Geometry check sheet. Reference: drawing and pictorial views, mm from the part's lowest x, y, z. A direction names the side the tool comes from. Coordinates: 2 decimals unless noted, no trailing zeros. Loops run counter-clockwise (first coordinate to the right, second up) from the corner with the lowest first, then second, coordinate; pieces in that order, holes last. Notation, with made-up numbers: (85, -23) - (139, -23) arc R16 ccw to (139, -10) - close; hole circle Ø11 at (16.5, -9.75). An arc over 180 degrees is marked (long way). Use a Markdown table: item, result. Add a question column.
1) Sectioned sample at A-A, the plane z = 7.75. Enter the section's corners in (x, y), then the cut area to 3 significant figures.
2) Thickness scan on line 1 (Y direction, x = 0.35, z = 8); line 2 (Z direction, x = 1.4, y = 17.75); line 3 (Z direction, x = 0.3, y = 5). Record the ranges inside material, lowest first.
3) Tool access check on the marked faces 1, 2, 3, 4 and 5. Record the directions out of +Z, -Z, +X, -X, +Y, -Y that give a thin tool (end or side, any length) a straight path to the whole face; none if there is none.
4) Go/stop test with flat-tipped pins: P1, Ø2.5, axis at x = 3.5, y = 14.5, coming from the -Z side; P2, Ø2.5, axis at x = 2, z = 12.5, coming from the -Y side. Record where each tip stops, or that it passes through.
5) Draft check along Y on the marked faces 6, 7 and 8. Enter one of: pulls with the +Y half, pulls with the -Y half, needs draft (parallel to the pull), parting line crosses it, or undercut.
6) Sectioned sample at D-D, the plane y = 5.25. Enter the section's corners in (x, z), then the cut area to 3 significant figures.
7) Sectioned sample at C-C, the plane z = 12.25. Enter the section's corners in (x, y).
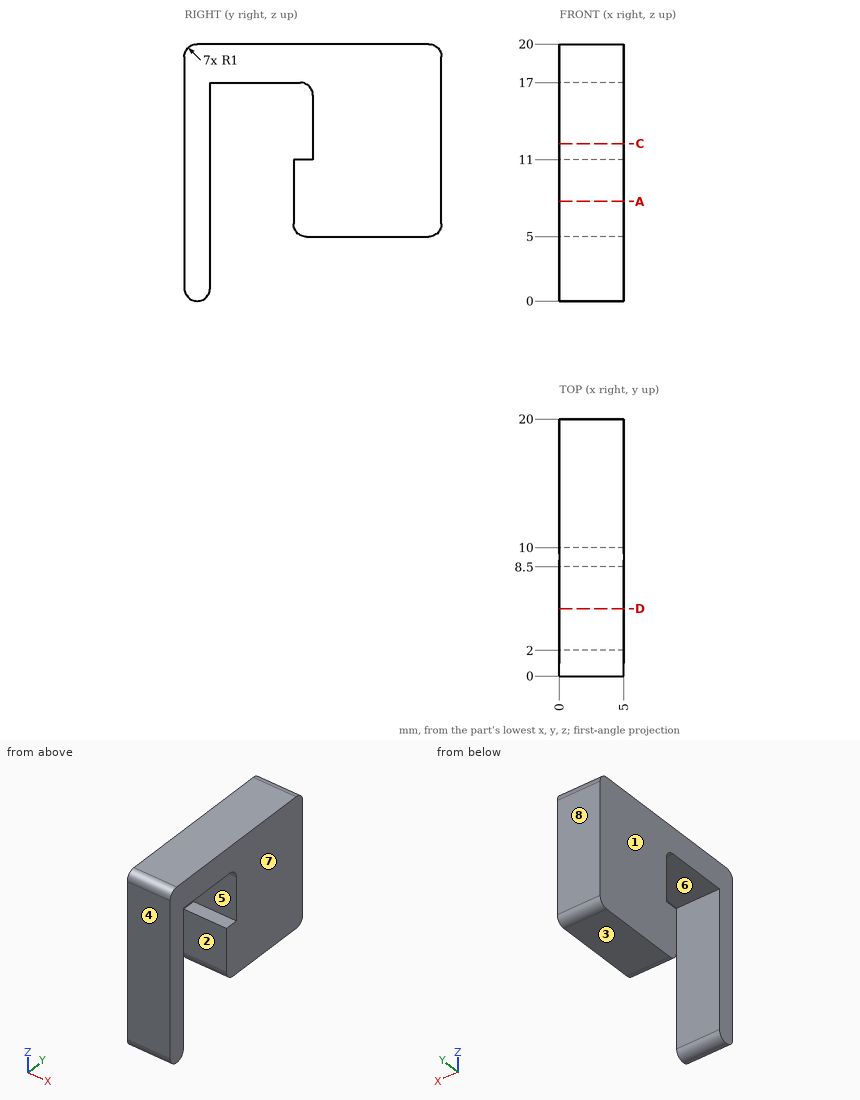
Solved:
| question | item | result |
|---|---|---|
| 1 | outline | (0, 0) - (5, 0) - (5, 2) - (0, 2) - close; (0, 8.5) - (5, 8.5) - (5, 20) - (0, 20) - close |
| 1 | area | 67.5 mm2 |
| 2 | line 1 | y = 0 to 2, 8.5 to 20 |
| 2 | line 2 | z = 5 to 20 |
| 2 | line 3 | z = 17 to 20 |
| 3 | face 1 | +Z, -Z, -X, +Y, -Y |
| 3 | face 2 | -Z, +X, -X |
| 3 | face 3 | -Z, +X, -X, +Y |
| 3 | face 4 | +Z, -Z, +X, -X, -Y |
| 3 | face 5 | +X, -X |
| 4 | P1 | stops at z = 5 |
| 4 | P2 | stops at y = 0 |
| 5 | face 6 | undercut |
| 5 | face 7 | needs draft |
| 5 | face 8 | pulls with the +Y half |
| 6 | outline | (0, 17) - (5, 17) - (5, 20) - (0, 20) - close |
| 6 | area | 15.0 mm2 |
| 7 | outline | (0, 0) - (5, 0) - (5, 2) - (0, 2) - close; (0, 10) - (5, 10) - (5, 20) - (0, 20) - close |
